from build123d import *

# Parameters (mm, degrees)
F0_W     = 90
F0_H     = 39.5
F1_DEPTH = 45
F2_R     = 5.25
F3_DEPTH = 39.5
F5_DEPTH = 45.001
F6_R     = 5


with BuildPart() as f1:
    # F0 (on Top) → F1 (new body)
    with BuildSketch(Plane.XY):
        Rectangle(F0_W, F0_H)
    extrude(amount=F1_DEPTH)

    # F2 (on face) → F3 (cut, through all)
    with BuildSketch(Plane.XZ.offset(19.75)):
        with Locations((0, 12.4)):
            Circle(F2_R)
    extrude(amount=-F3_DEPTH, mode=Mode.SUBTRACT)

    # F4 (on face) → F5 (cut, through all)
    with BuildSketch(Plane.XY.offset(45)):
        Polygon((25.5, 6.25), (0, 6.25), (-25.5, 6.25), (-25.5, 0.25), (0, 0.25), (25.5, 0.25), align=None)
    extrude(amount=-F5_DEPTH, mode=Mode.SUBTRACT)

    # F6
    f6_edges = [f1.edges().sort_by_distance(p)[0] for p in [
        (-45, -19.75, 22.5),
        (45, -19.75, 22.5),
    ]]
    fillet(f6_edges, radius=F6_R)


solid = f1.part
Design review of the part built by this model. Coordinates are the model's own, in mm. A direction names the side the tool comes from. Give positions to 0.01 mm unless a question says otherwise; leave off trailing zeros. Loops run counter-clockwise (first coordinate to the right, second up) from the corner with the lowest first, then second, coordinate; pieces in that order, holes last. Notation, with made-up numbers: (-25, -18) - (-20, -18) arc R31 ccw to (-20, 17) - close; hole circle Ø3 at (39.25, 65.5). An arc over 180 degrees is marked (long way). Use CSV: the item, a comma, the result in double quotes. Start each with the question number.
1. Add section C-C (y = 1.5). State the section outline as (x, z) points.
2. Wall thickness on L1, parallel to X at y = -10, z = 12; L2, parallel to Y at x = 24.5, z = 5.5; L3, parallel to Z at x = 0, y = 15.5: over which ranges is each line inside the solid? List them lowest first.
3. Draft analysis for pull direction X (two halves, no side actions). For faces 3 (the flat face through (45, 2, 22)), 4 (the flat face through (-45, 2, 22)), 5 (the flat face through (-1, 19.75, 22)), 6 (the flat face through (0, 6.25, 23)), state which applies: released by +X, released by -X, zero draft, split by the parting line, or undercut.
4. Machinability: for faces 1 (the flat face through (0, 0.25, 23)), 2 (the cylindrical face through (-0.683, 12.906, 17.605)), which of the approach directions +Z, -Z, +X, -X, +Y, -Y give a long, thin tool a straight path to every point of the face, cutting with its end or side? Answer none if there is none.
5. Add section A-A (z = 31). State the section outline as (x, y) points.
6. Add section D-D (z = 12.4). State the section outline as (x, y) points.
7. Add section B-B (x = -6.5). State the section outline as (y, z) points, plus the area to 3 significant figures.
8. Insertion check: P1, Ø12, axis at x = 2, z = 8, coming from the -Y side; P2, Ø1.5, axis at x = 23.5, y = 5, coming from the +Z side. Each pin has a flat end and moves straight along its axis. Give the tip position at first contact, or say it passes through.
Results found:
1,outline,"(-45, 0) - (-25.5, 0) - (-25.5, 45) - (-45, 45) - close; (25.5, 0) - (45, 0) - (45, 45) - (25.5, 45) - close"
2,L1,"x = -45 to -5.23, 5.23 to 45"
2,L2,"y = -19.75 to 0.25, 6.25 to 19.75"
2,L3,"z = 0 to 7.15, 17.65 to 45"
3,face 3,"released by +X"
3,face 4,"released by -X"
3,face 5,"zero draft"
3,face 6,"undercut"
4,face 1,"+Z, -Z"
4,face 2,"+Y, -Y"
5,outline,"(-45, -14.75) arc R5 ccw to (-40, -19.75) - (40, -19.75) arc R5 ccw to (45, -14.75) - (45, 19.75) - (-45, 19.75) - close; hole (-25.5, 0.25) - (25.5, 0.25) - (25.5, 6.25) - (-25.5, 6.25) - close"
6,outline,"(-45, -14.75) arc R5 ccw to (-40, -19.75) - (-5.25, -19.75) - (-5.25, 0.25) - (-25.5, 0.25) - (-25.5, 6.25) - (-5.25, 6.25) - (-5.25, 19.75) - (-45, 19.75) - close; (5.25, -19.75) - (40, -19.75) arc R5 ccw to (45, -14.75) - (45, 19.75) - (5.25, 19.75) - (5.25, 6.25) - (25.5, 6.25) - (25.5, 0.25) - (5.25, 0.25) - close"
7,outline,"(-19.75, 0) - (0.25, 0) - (0.25, 45) - (-19.75, 45) - close; (6.25, 0) - (19.75, 0) - (19.75, 45) - (6.25, 45) - close"
7,area,"1,510 mm²"
8,P1,"stops at y = -19.75"
8,P2,"passes through"
